CAD build for the part. Positions are in the model's coordinates, mm. Face numbers are marked on the shaded views. A direction names the side the tool comes from. Round coordinates to 2 decimals unless told otherwise and drop trailing zeros. Loops run counter-clockwise (first coordinate to the right, second up) from the corner with the lowest first, then second, coordinate; pieces in that order, holes last. Notation, with made-up numbers: M 57,-20 L 106,-20 A14 cw 106,-8 Z; hole C 21.25,-13.75 d8. An arc over 180 degrees is marked long. Use one line per item in the form item = value.
Autodesk Inventor part; units mm, degrees
ref_plane "Work Plane1" through (0, 9, 0) normal (0, 1, 0) x (-1, 0, 0)
ref_plane "YZ Plane" through (0, 0, 0) normal (1, 0, 0) x (0, 1, 0)
ref_plane "XY Plane" through (0, 0, 0) normal (0, 0, 1) x (1, 0, 0)
sketch "Sketch1" plane through (0, 0, 0) normal (0, 0, 1) x (1, 0, 0)
  circle A0 centre (0, 0) radius 7
extrude "Extrusion1" add sketch "Sketch1" against normal blind 35
sketch "Sketch2" plane through (0, 0, 0) normal (0, 0, 1) x (1, 0, 0)
  circle A0 centre (0, 0) radius 7
  circle A1 centre (0, 0) radius 5.25
extrude "Extrusion2" cut sketch "Sketch2" against normal blind 5 contours A1
sketch "Sketch3" plane through (0, 0, -5) normal (0, 0, 1) x (1, 0, 0)
  circle A0 centre (0, 0) radius 5.25
  circle A1 centre (0, 0) radius 1.5
extrude "Extrusion3" cut sketch "Sketch3" against normal blind 30 contours A1
sketch "Sketch4" plane through (0, 0, -35) normal (0, 0, -1) x (-1, 0, 0)
  circle A0 centre (0, 0) radius 1.5
  circle A1 centre (0, 0) radius 7
  circle A2 centre (0, 0) radius 1.5
  circle A3 centre (0, 0) radius 3
extrude "Extrusion4" cut sketch "Sketch4" against normal blind 9 contours A3
ref_plane "Work Plane1" through (0, 9, 0) normal (0, 1, 0) x (-1, 0, 0)
sketch "Sketch5" plane through (0, 9, 0) normal (0, 1, 0) x (-1, 0, 0)
  line L0 (3, -35) -> (-3, -35)
  line L1 (-7, -35) -> (7, -35)
  circle A0 centre (0, -29) radius 1.5
  point P0 (0, 0)
extrude "Extrusion5" cut sketch "Sketch5" against normal blind 9
thread "Thread1"
fillet "Fillet1" radius 0.4 1 edges at (-7, 0, -35)
properties part number "Shaft"
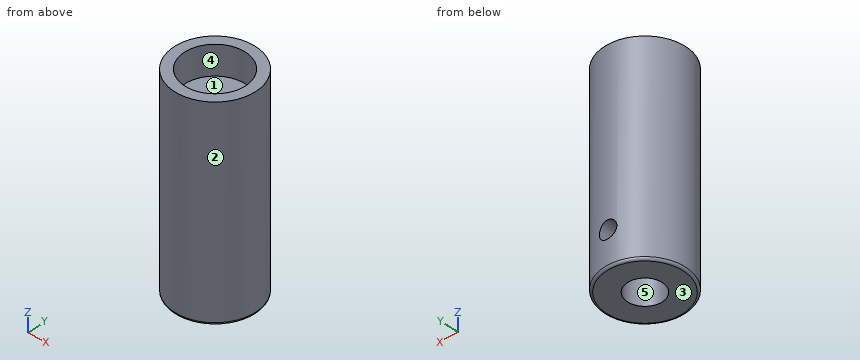
1. Drop flat-ended pins along their axis: P1, Ø1.5, axis at x = 4.5, z = -21.5, coming from the -Y side; P2, Ø1.5, axis at y = -3, z = -20.5, coming from the +X side; P3, Ø2, axis at y = -2, z = -6.5, coming from the -X side. Give the stop position or say it passes through.
Completed:
P1 = -5.91
P2 = 6.63
P3 = -6.93
2. Probe line 1 along Y through (x, z) = (0, -3.05); line 2 along Y through (x, z) = (0, -20); line 3 along Z through (x, y) = (0, 4.85). List the from-to ranges inside material, lowest first. Write a range as from..to.
Completed:
line_1 = -7..-5.25, 5.25..7
line_2 = -7..-1.5, 1.5..7
line_3 = -35..-30.5, -27.5..-5
3. Cut at C-C on z = -8.5. Write the cut outline in (x, y), and give its area (3 significant figures).
Completed:
outline = C 0,0 d14; hole C 0,0 d3
area = 147 mm2
4. Cut at A-A on y = 0. Write the cut outline in (x, z).
Completed:
outline = M -7,-34.6 A0.4 ccw -6.6,-35 L -3,-35 L -3,-26 L -1.5,-26 L -1.5,-5 L -5.25,-5 L -5.25,0 L -7,0 Z; M 1.5,-26 L 3,-26 L 3,-35 L 6.6,-35 A0.4 ccw 7,-34.6 L 7,0 L 5.25,0 L 5.25,-5 L 1.5,-5 Z
5. Cut at B-B on x = 0. Write the cut outline in (y, z).
Completed:
outline = M -7,-34.6 A0.4 ccw -6.6,-35 L -3,-35 L -3,-26 L -1.5,-26 L -1.5,-5 L -5.25,-5 L -5.25,0 L -7,0 Z; M 1.5,-26 L 3,-26 L 3,-27.5 L 7,-27.5 L 7,0 L 5.25,0 L 5.25,-5 L 1.5,-5 Z; M 3,-35 L 6.6,-35 A0.4 ccw 7,-34.6 L 7,-30.5 L 3,-30.5 Z
6. Cut at D-D on z = -29. Write the cut outline in (x, y).
Completed:
outline = M -1.5,2.6 L -1.5,6.84 A7 ccw long 1.5,6.84 L 1.5,2.6 A3 cw long Z
7. Tool access for the marked faces 4 and 5: list every direction of +Z, -Z, +X, -X, +Y, -Y with a clear straight run to the whole face (end or side of a thin tool).
Completed:
face_4 = +Z
face_5 = -Z
8. Pull direction X, two halves, no side cores. Call the marked faces 1, 2 and 3: +X half, -X half, draft (parallel to the pull), parting line (faces both ways), or undercut.
Completed:
face_1 = undercut
face_2 = parting line
face_3 = draft
